```python
from build123d import *

# Parameters (mm, degrees)
BASE_FLANGE1_DEPTH       = 0.7
EDGE_FLANGE1_START       = -2.45
EDGE_FLANGE1_DEPTH       = 4.9
EDGE_FLANGE1_START_2     = -2.8
EDGE_FLANGE1_2_OUTLINE_W = 0.7
EDGE_FLANGE1_2_OUTLINE_H = 0.05
EDGE_FLANGE1_2_DEPTH     = 0.35
EDGE_FLANGE1_START_3     = 2.45
EDGE_FLANGE1_3_OUTLINE_W = 0.7
EDGE_FLANGE1_3_OUTLINE_H = 0.05
EDGE_FLANGE1_3_DEPTH     = 0.35
EDGE_FLANGE1_4_DEPTH     = 4.9
CUT_EXTRUDE1_DEPTH       = 10
SKETCH10_R               = 1
BOSS_EXTRUDE1_DEPTH      = 1
BOSS_EXTRUDE1_DRAFT      = -17
CUT_EXTRUDE2_DEPTH       = 10.571050099
CHAMFER1_SIZE            = 1
M3_TAPPED_HOLE1_D        = 2.5
M3_TAPPED_HOLE1_DEPTH    = 7.5
M3_TAPPED_HOLE1_TIP      = 0.751075774


# Read off the part's stored shape, not the designer's step: Edge-Flange1
# Sheet-metal steps are written as plain solids
with BuildPart() as part:
    # Sketch1 → Base-Flange1 (new body)
    with BuildSketch(Plane(origin=(0, 0, 0), x_dir=(1, 0, 0), z_dir=(0, 1, 0))):
        Polygon((-2.45, -3.25), (-3.5, -3.25), (-3.5, 3.25), (3.5, 3.25), (3.5, -3.25), (2.45, -3.25), (2.45, -4.75), (-2.45, -4.75), align=None)
    extrude(amount=-BASE_FLANGE1_DEPTH)

    # Edge-Flange1 outline → Edge-Flange1 (cut)
    with BuildSketch(Plane.YZ.offset(EDGE_FLANGE1_START)):
        with BuildLine():
            Line((-0.7, 4.75), (-0.7, 3.55))
            ThreePointArc((-0.7, 3.55), (-0.509950493, 4.198074069), (0, 4.640871211))
            Line((0, 4.640871211), (0, 4.75))
            Line((0, 4.75), (-0.7, 4.75))
        make_face()
    extrude(amount=EDGE_FLANGE1_DEPTH, mode=Mode.SUBTRACT)

    # Edge-Flange1 2 outline → Edge-Flange1 2 (cut)
    with BuildSketch(Plane.YZ.offset(EDGE_FLANGE1_START_2)):
        with Locations((-0.35, 3.225)):
            Rectangle(EDGE_FLANGE1_2_OUTLINE_W, EDGE_FLANGE1_2_OUTLINE_H)
    extrude(amount=EDGE_FLANGE1_2_DEPTH, mode=Mode.SUBTRACT)

    # Edge-Flange1 3 outline → Edge-Flange1 3 (cut)
    with BuildSketch(Plane.YZ.offset(EDGE_FLANGE1_START_3)):
        with Locations((-0.35, 3.225)):
            Rectangle(EDGE_FLANGE1_3_OUTLINE_W, EDGE_FLANGE1_3_OUTLINE_H)
    extrude(amount=EDGE_FLANGE1_3_DEPTH, mode=Mode.SUBTRACT)

    # Edge-Flange1 4 outline → Edge-Flange1 4 (add)
    with BuildSketch(Plane.YZ.offset(EDGE_FLANGE1_START)):
        with BuildLine():
            Line((0, 4.640871211), (0, 3.55))
            ThreePointArc((0, 3.55), (0.146446609, 3.903553391), (0.5, 4.05))
            Line((0.5, 4.05), (5.8, 4.05))
            Line((5.8, 4.05), (5.8, 4.75))
            Line((5.8, 4.75), (0.5, 4.75))
            ThreePointArc((0.5, 4.75), (0.244114727, 4.722400412), (0, 4.640871211))
        make_face()
    extrude(amount=EDGE_FLANGE1_4_DEPTH)

    # Sketch9 → Cut-Extrude1 (cut)
    with BuildSketch(Plane(origin=(0, 0, 4.05), x_dir=(-1, 0, 0), z_dir=(0, 0, -1))):
        with BuildLine():
            ThreePointArc((0, 5.8), (1.732411614, 5.082411614), (2.45, 3.35))
            Line((2.45, 3.35), (2.45, 5.8))
            Line((2.45, 5.8), (0, 5.8))
        make_face()
        with BuildLine():
            ThreePointArc((-2.45, 3.35), (-1.732411614, 5.082411614), (0, 5.8))
            Line((0, 5.8), (-2.45, 5.8))
            Line((-2.45, 5.8), (-2.45, 3.35))
        make_face()
    extrude(amount=-CUT_EXTRUDE1_DEPTH, mode=Mode.SUBTRACT)


with BuildPart() as boss_extrude1_tool:
    # Sketch10 → Boss-Extrude1 (with draft: the straight prism first)
    with BuildSketch(Plane(origin=(0, 0, 4.05), x_dir=(-1, 0, 0), z_dir=(0, 0, -1))):
        with Locations((0, 3.35)):
            Circle(SKETCH10_R)
    extrude(amount=BOSS_EXTRUDE1_DEPTH)
    # Boss-Extrude1: the draft: its side faces are tilted about the plane it starts from
    boss_extrude1_sides = [boss_extrude1_tool.faces().sort_by_distance(p)[0] for p in [
        (1, 3.35, 3.55),
    ]]
    draft(boss_extrude1_sides, Plane(origin=(0, 0, 4.05), x_dir=(-1, 0, 0), z_dir=(0, 0, -1)), BOSS_EXTRUDE1_DRAFT)


with BuildPart() as part_1:
    add(part.part)

    # Boss-Extrude1: add boss_extrude1_tool
    add(boss_extrude1_tool.part)

    # Sketch11 → Cut-Extrude2 (cut, through all)
    with BuildSketch(Plane(origin=(2.45, 0, 0), x_dir=(0, 0, -1), z_dir=(1, 0, 0))):
        Polygon((-3.254043784, 4.795439766), (-2.944980446, 4.391765202), (-3.304503105, 4.000705467), (-2.944980446, 3.584416072), (-3.254043784, 3.073515451), (-2.961297011, 2.691152319), (-3.254043784, 2.43832556), (-2.961297011, 2.261231833), (-3.304503105, 1.887919941), (-2.402542749, 1.887919941), (-2.522383636, 4.908973238), align=None)
    extrude(amount=-CUT_EXTRUDE2_DEPTH, mode=Mode.SUBTRACT)

    # Chamfer1
    chamfer1_edges = [part_1.edges().sort_by_distance(p)[0] for p in [
        (-3.5, -0.35, -3.25),
        (3.5, -0.35, -3.25),
    ]]
    chamfer(chamfer1_edges, length=CHAMFER1_SIZE)

    # M3 Tapped Hole1
    with Locations(Plane(origin=(0, -0.7, 0), x_dir=(-1, 0, 0), z_dir=(0, -1, 0))):
        with Locations((0, 0)):
            Hole(M3_TAPPED_HOLE1_D / 2, depth=M3_TAPPED_HOLE1_DEPTH)
            with Locations((0, 0, -(M3_TAPPED_HOLE1_DEPTH + M3_TAPPED_HOLE1_TIP / 2))):  # 118° drill point
                Cone(0, M3_TAPPED_HOLE1_D / 2, M3_TAPPED_HOLE1_TIP, mode=Mode.SUBTRACT)


solid = part_1.part
```
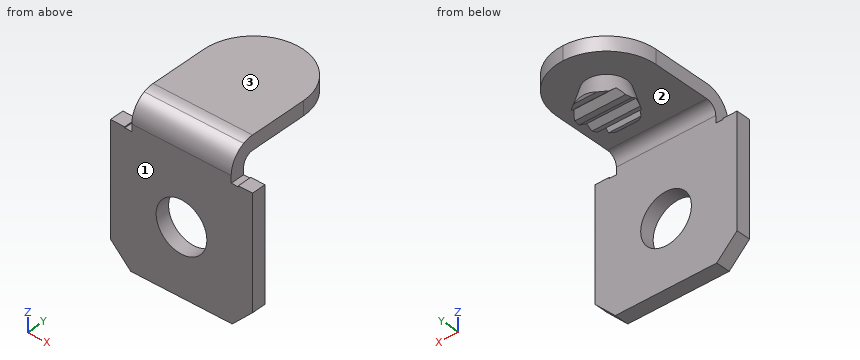
Read the model definition and answer for the solid it produces. Units are mm, in the model's axes. Face numbers are marked on the shaded views. Coordinates: 2 decimals unless noted, no trailing zeros. Write each loop counter-clockwise with the first axis right and the second up, starting at its lowest first coordinate (ties: lowest second). Pieces come first, ordered by that corner, then holes. Notation, with made-up numbers: (86, 6) -> (132, 6) arc R19 ccw to (132, 11) -> close; hole circle Ø10 at (-36.5, 13). An arc over 180 degrees is marked (long way). Return JSON: item names as keys, results as strings.
1. A cutting plane is placed at D-D (y = 1). Determine the outline of the cut face in (x, z).
Found:
{"outline": "(-2.45, 4.05) -> (2.45, 4.05) -> (2.45, 4.75) -> (-2.45, 4.75) -> close"}
2. Each of these flat-tipped pins is pushed along its axis until it touches: P1, Ø1.5, axis at x = 0, z = 0, coming from the +Y side; P2, Ø1.5, axis at x = 0.5, y = 4, coming from the -Z side; P3, Ø0.6, axis at x = 3, y = 0, coming from the +Z side; P4, Ø1.2, axis at y = 0.5, z = 4, coming from the +X side. Where does it stop, or does it pass through?
Found:
{"P1": "through", "P2": "z = 3.05", "P3": "z = 3.25", "P4": "x = 2.45"}
3. A cutting plane is placed at C-C (z = -0.75). Determine the outline of the cut face in (x, y), and give its area (3 significant figures).
Found:
{"outline": "(-3.5, -0.7) -> (-1, -0.7) -> (-1, 0) -> (-3.5, 0) -> close; (1, -0.7) -> (3.5, -0.7) -> (3.5, 0) -> (1, 0) -> close", "area": "3.50 mm2"}
4. Find the intervals of material crossed by line 1 along Y through (x, z) = (-2.25, -1); line 2 along Z through (x, y) = (0, -0.2); line 3 along Z through (x, y) = (0, -0.45), in increasing order. Write a range as from..to.
Found:
{"line 1": "-0.7..0", "line 2": "-3.25..-1.25, 1.25..4.52", "line 3": "-3.25..-1.25, 1.25..4.28"}
5. Determine the mould class of the marked faces 1, 2 and 3 for opening direction Y: pulls with the +Y half, pulls with the -Y half, needs draft (parallel to the pull), parting line crosses it, or undercut.
Found:
{"face 1": "pulls with the -Y half", "face 2": "undercut", "face 3": "needs draft"}
6. A cutting plane is placed at B-B (x = -2). Determine the outline of the cut face in (y, z), and give its area (3 significant figures).
Found:
{"outline": "(-0.7, -3.25) -> (0, -3.25) -> (0, 3.55) arc R0.5 cw to (0.5, 4.05) -> (4.77, 4.05) -> (4.77, 4.75) -> (0.5, 4.75) arc R1.2 ccw to (-0.7, 3.55) -> close", "area": "8.68 mm2"}
7. A cutting plane is placed at A-A (z = 1). Determine the outline of the cut face in (x, y), and give its area (3 significant figures).
Found:
{"outline": "(-3.5, -0.7) -> (-0.75, -0.7) -> (-0.75, 0) -> (-3.5, 0) -> close; (0.75, -0.7) -> (3.5, -0.7) -> (3.5, 0) -> (0.75, 0) -> close", "area": "3.85 mm2"}
